from build123d import *

# Parameters (mm, degrees)
SKETCH1_R           = 1.5
BOSS_EXTRUDE1_DEPTH = 2.8
CUT_EXTRUDE1_REACH  = 4.8
SKETCH2_R           = 1.5
CUT_EXTRUDE2_REACH  = 4.8
SKETCH3_R           = 10.5
CUT_EXTRUDE3_REACH  = 4.8
SKETCH4_R           = 5
FILLET1_R           = 1


with BuildPart() as part:
    # Sketch1 → Boss-Extrude1 (new body)
    with BuildSketch(Plane(origin=(0, 0, 0), x_dir=(1, 0, 0), z_dir=(0, 1, 0))):
        Polygon((-76, -79.75), (56, -79.75), (56, -38.75), (76, -38.75), (76, 79.75), (-56, 79.75), (-56, 49.75), (-76, 49.75), align=None)
        with Locations((-46, -66.75)):
            Circle(SKETCH1_R, mode=Mode.SUBTRACT)
        with Locations((-66, -29.75)):
            Circle(SKETCH1_R, mode=Mode.SUBTRACT)
        with Locations((41, -66.75)):
            Circle(SKETCH1_R, mode=Mode.SUBTRACT)
        with Locations((66, -18.75)):
            Circle(SKETCH1_R, mode=Mode.SUBTRACT)
        with Locations((66, 59.75)):
            Circle(SKETCH1_R, mode=Mode.SUBTRACT)
    extrude(amount=BOSS_EXTRUDE1_DEPTH)

    # Sketch2 → Cut-Extrude1 (cut, up to next)
    with BuildSketch(Plane(origin=(0, 2.8, 0), x_dir=(1, 0, 0), z_dir=(0, 1, 0)), mode=Mode.PRIVATE) as cut_extrude1_sk1:
        with Locations((31, -44.75)):
            Circle(SKETCH2_R)
    cut_extrude1_tool1 = extrude(cut_extrude1_sk1.sketch, amount=-CUT_EXTRUDE1_REACH, mode=Mode.PRIVATE) & part.part
    add(cut_extrude1_tool1.solids().sort_by_distance((31, 2.8, 44.75))[0], mode=Mode.SUBTRACT)
    # Sketch2 → Cut-Extrude1 (cut, up to next)
    with BuildSketch(Plane(origin=(0, 2.8, 0), x_dir=(1, 0, 0), z_dir=(0, 1, 0)), mode=Mode.PRIVATE) as cut_extrude1_sk2:
        with Locations((-6.118257487, -10.040707856)):
            Circle(SKETCH2_R)
    cut_extrude1_tool2 = extrude(cut_extrude1_sk2.sketch, amount=-CUT_EXTRUDE1_REACH, mode=Mode.PRIVATE) & part.part
    add(cut_extrude1_tool2.solids().sort_by_distance((-6.118257, 2.8, 10.040708))[0], mode=Mode.SUBTRACT)
    # Sketch2 → Cut-Extrude1 (cut, up to next)
    with BuildSketch(Plane(origin=(0, 2.8, 0), x_dir=(1, 0, 0), z_dir=(0, 1, 0)), mode=Mode.PRIVATE) as cut_extrude1_sk3:
        with Locations((-17.618257487, -29.959292144)):
            Circle(SKETCH2_R)
    cut_extrude1_tool3 = extrude(cut_extrude1_sk3.sketch, amount=-CUT_EXTRUDE1_REACH, mode=Mode.PRIVATE) & part.part
    add(cut_extrude1_tool3.solids().sort_by_distance((-17.618257, 2.8, 29.959292))[0], mode=Mode.SUBTRACT)

    # Sketch3 → Cut-Extrude2 (cut, up to next)
    with BuildSketch(Plane(origin=(0, 2.8, 0), x_dir=(1, 0, 0), z_dir=(0, 1, 0)), mode=Mode.PRIVATE) as cut_extrude2_sk1:
        with Locations((-36, -42.75)):
            Circle(SKETCH3_R)
    cut_extrude2_tool1 = extrude(cut_extrude2_sk1.sketch, amount=-CUT_EXTRUDE2_REACH, mode=Mode.PRIVATE) & part.part
    add(cut_extrude2_tool1.solids().sort_by_distance((-36, 2.8, 42.75))[0], mode=Mode.SUBTRACT)

    # Sketch4 → Cut-Extrude3 (cut, up to next)
    with BuildSketch(Plane(origin=(0, 2.8, 0), x_dir=(1, 0, 0), z_dir=(0, 1, 0)), mode=Mode.PRIVATE) as cut_extrude3_sk1:
        with Locations((-76, -16.75)):
            Circle(SKETCH4_R)
    cut_extrude3_tool1 = extrude(cut_extrude3_sk1.sketch, amount=-CUT_EXTRUDE3_REACH, mode=Mode.PRIVATE) & part.part
    add(cut_extrude3_tool1.solids().sort_by_distance((-76, 2.8, 16.75))[0], mode=Mode.SUBTRACT)

    # Fillet1
    fillet1_edges = [part.edges().sort_by_distance(p)[0] for p in [
        (-76, 1.4, 21.75),
        (-76, 1.4, 11.75),
    ]]
    fillet(fillet1_edges, radius=FILLET1_R)


solid = part.part
Work out the finished part from the listing and answer in its coordinate system (mm). Round coordinates to 2 decimals unless told otherwise and drop trailing zeros. Write each loop counter-clockwise with the first axis right and the second up, starting at its lowest first coordinate (ties: lowest second). Pieces come first, ordered by that corner, then holes.
1) Given pin 1 Ø1.4 at (x, y) = (67.5, 2) entering from +Z; pin 2 Ø0.8 at (y, z) = (2, -70) entering from -X, each flat-ended and moving along its own axis, determine where each tip first touches the part or whether it passes through.
2) A cutting plane is placed at B-B (y = 0.5). Give the number of separate pieces and of enclosed holes in the cut face, plus the area to 3 significant figures.
3) Straight lines are drawn through the part: line 1 (X direction, y = 1.4, z = 66.75); line 2 (Z direction, x = 66, y = 2.25); line 3 (Z direction, x = -36, y = 0.9). For each, find the intervals that lie inside material, in ascending order.
4) A cutting plane is placed at A-A (z = -53). Give the vertices of the cut face in (x, y), plus the area to 3 significant figures.
5) The mould has two halves that part along Z. Classify faces 1 (the flat face through (-1, 2.8, -1)), 2 (the cylindrical face through (-46.49, 1.42, 42.29)): pulls with the +Z half, pulls with the -Z half, needs draft (parallel to the pull), parting line crosses it, or undercut.
6) A cutting plane is placed at C-C (z = 14). Give the vertices of the cut face in (x, y).
Completed:
1. pin 1: stops at z = 38.75
1. pin 2: stops at x = -56
2. separate pieces: 1
2. enclosed holes: 9
2. area: 22,400 mm2
3. line 1: x = -76 to -47.5, -44.5 to 39.5, 42.5 to 56
3. line 2: z = -79.75 to -61.25, -58.25 to 17.25, 20.25 to 38.75
3. line 3: z = -79.75 to 32.25, 53.25 to 79.75
4. outline: (-56, 0) - (76, 0) - (76, 2.8) - (-56, 2.8) - close
4. area: 370 mm2
5. face 1: needs draft
5. face 2: undercut
6. outline: (-71.82, 0) - (76, 0) - (76, 2.8) - (-71.82, 2.8) - close
